Read the model definition and answer for the solid it produces. Units are mm, in the model's axes. A direction names the side the tool comes from. Give positions to 0.01 mm unless a question says otherwise; leave off trailing zeros. Loops run counter-clockwise (first coordinate to the right, second up) from the corner with the lowest first, then second, coordinate; pieces in that order, holes last.
(1) Straight lines are drawn through the part: probe 1 along X at (y, z) = (-58, 23); probe 2 along Z at (x, y) = (-60.5, -30); probe 3 along X at (y, z) = (15, 36.5). For each, find the intervals that lie inside material, in ascending order.
(2) Each of these flat-tipped pins is pushed along its axis until it touches: P1, Ø20, axis at x = -39.5, y = 27.5, coming from the +Z side; P2, Ø16, axis at y = -70.33, z = 27, coming from the -X side; P3, Ø16, axis at y = -67.5, z = 33, coming from the +X side; P4, Ø20, axis at x = -39, y = 23, coming from the -Z side. Where does it stop, or does it pass through?
(3) Find section D-D, the plane y = 10. Write down the section's boundary in (x, z), then the cut area to 3 significant figures.
(4) Find section B-B, the plane y = -39.5. Write down the section's boundary in (x, z).
(5) Which of the six approach directions +Z, -Z, +X, -X, +Y, -Y give full straight-line access (tool end or side, diameter ignored) to faces 1 (the face through (-24.833, 28, 27)), 2 (the face through (-38, 28, 14.5)), 3 (the face through (-38, 28, 39.5)), 4 (the face through (-34, 42.667, 18)), 5 (the face through (-49.833, 28, 27))?
(6) Find section C-C, the plane z = 50.5. Write down the section's boundary in (x, y).
(7) Find section A-A, the plane z = 27. State how many separate pieces and enclosed holes the cut face has, then the cut area to 3 significant figures.
```python
from build123d import *

# Parameters (mm, degrees)
SKETCH1_W           = 56
SKETCH1_H           = 140
BOSS_EXTRUDE1_DEPTH = 54
CUT_EXTRUDE4_DEPTH  = 54
SKETCH5_OUTSIDE_W   = 88.032
SKETCH5_OUTSIDE_H   = 174.032
SKETCH5_OUTSIDE_R   = 9
CUT_EXTRUDE6_DEPTH  = 60
SKETCH6_OUTSIDE_W   = 90.032
SKETCH6_OUTSIDE_H   = 88.032
SKETCH6_OUTSIDE_W_2 = 25
SKETCH6_OUTSIDE_H_2 = 25
CUT_EXTRUDE7_DEPTH  = 30
SKETCH7_R           = 9
BOSS_EXTRUDE2_DEPTH = 20


with BuildPart() as part:
    # Sketch1 → Boss-Extrude1 (new body)
    with BuildSketch(Plane.XY):
        with Locations((-37.333333333, -27.333333333)):
            Rectangle(SKETCH1_W, SKETCH1_H)
    extrude(amount=BOSS_EXTRUDE1_DEPTH)

    # Sketch2 → Cut-Extrude4 (cut)
    with BuildSketch(Plane.XY.offset(54)):
        with BuildLine():
            Line((-52.333333333, 6.259015594), (-52.333333333, 42.666666667))
            Line((-52.333333333, 42.666666667), (-65.333333333, 42.666666667))
            Line((-65.333333333, 42.666666667), (-65.333333333, -30.333333244))
            ThreePointArc((-65.333333333, -30.333333244), (-63.717759237, -20.959856403), (-59.057471264, -12.668061438))
            ThreePointArc((-59.057471264, -12.668061438), (-54.064305564, -3.783995357), (-52.333333333, 6.259015594))
        make_face()
        with BuildLine():
            Line((-37.333333333, -97.333333333), (-37.333333333, -18.333333333))
            ThreePointArc((-37.333333333, -18.333333333), (-47.23282827, -22.433838397), (-51.333333333, -32.333333333))
            Line((-51.333333333, -32.333333333), (-51.333333333, -54.582044639))
            Line((-51.333333333, -54.582044639), (-51.333333333, -97.333333333))
            Line((-51.333333333, -97.333333333), (-37.333333333, -97.333333333))
        make_face()
        with BuildLine():
            ThreePointArc((-37.333333333, -18.333333333), (-27.433838397, -22.433838397), (-23.333333333, -32.333333333))
            Line((-23.333333333, -32.333333333), (-23.333333333, -97.333333333))
            Line((-23.333333333, -97.333333333), (-9.333333333, -97.333333333))
            Line((-9.333333333, -97.333333333), (-9.333333333, 42.666666667))
            Line((-9.333333333, 42.666666667), (-22.333333333, 42.666666667))
            Line((-22.333333333, 42.666666667), (-37.333333333, 42.666666667))
            Line((-37.333333333, 42.666666667), (-37.333333333, -18.333333333))
        make_face()
        with BuildLine():
            Line((-23.333333333, -97.333333333), (-23.333333333, -32.333333333))
            ThreePointArc((-23.333333333, -32.333333333), (-27.433838397, -22.433838397), (-37.333333333, -18.333333333))
            Line((-37.333333333, -18.333333333), (-37.333333333, -97.333333333))
            Line((-37.333333333, -97.333333333), (-23.333333333, -97.333333333))
        make_face()
    extrude(amount=-CUT_EXTRUDE4_DEPTH, mode=Mode.SUBTRACT)

    # Mirror3: part across plane


with BuildPart() as part_1:
    add(part.part)
    add(part.part.mirror(Plane.ZY.offset(37.333333333)))

    # Sketch5 outside → Cut-Extrude6 (cut)
    # profile 1 of 2: a face of its own
    with BuildSketch(Plane(origin=(-9.333333333, 0, 0), x_dir=(0, 0, -1), z_dir=(1, 0, 0))):
        with Locations((-27, -27.333)):
            Rectangle(SKETCH5_OUTSIDE_W, SKETCH5_OUTSIDE_H)
        with BuildLine():
            Line((-42, 42.666666667), (-12, 42.666666667))
            Line((-12, 42.666666667), (-12, -35.347621964))
            ThreePointArc((-12, -35.347621964), (-10.377159088, -45.080907232), (-5.684210526, -53.761154264))
            ThreePointArc((-5.684210526, -53.761154264), (-27, -97.333333333), (-48.315789474, -53.761154264))
            ThreePointArc((-48.315789474, -53.761154264), (-43.622840912, -45.080907232), (-42, -35.347621964))
            Line((-42, -35.347621964), (-42, 42.666666667))
        make_face(mode=Mode.SUBTRACT)
    # profile 2 of 2: a face of its own
    with BuildSketch(Plane(origin=(-9.333333333, 0, 0), x_dir=(0, 0, -1), z_dir=(1, 0, 0))):
        with Locations(Location((-27, -70.333333333, 0), (0, 0, 90))):
            Circle(SKETCH5_OUTSIDE_R)
    extrude(amount=-CUT_EXTRUDE6_DEPTH, mode=Mode.SUBTRACT)

    # Sketch6 outside → Cut-Extrude7 (cut)
    with BuildSketch(Plane(origin=(0, 42.666666667, 0), x_dir=(1, 0, 0), z_dir=(0, 1, 0))):
        with Locations((-37.333, -27)):
            Rectangle(SKETCH6_OUTSIDE_W, SKETCH6_OUTSIDE_H)
        with Locations((-37.333333333, -27)):
            Rectangle(SKETCH6_OUTSIDE_W_2, SKETCH6_OUTSIDE_H_2, mode=Mode.SUBTRACT)
    extrude(amount=-CUT_EXTRUDE7_DEPTH, mode=Mode.SUBTRACT)

    # Sketch7 → Boss-Extrude2 (add)
    with BuildSketch(Plane(origin=(0, 42.666666667, 0), x_dir=(1, 0, 0), z_dir=(0, 1, 0))):
        with Locations(Location((-37.333333333, -27, 0), (0, 0, 270))):
            Circle(SKETCH7_R)
    extrude(amount=BOSS_EXTRUDE2_DEPTH)


solid = part_1.part
```
Entries:
1. probe 1: x = -65.33 to -51.33, -23.33 to -9.33
1. probe 2: z = 12 to 42
1. probe 3: x = -49.83 to -24.83
2. P1: stops at z = 39.5
2. P2: passes through
2. P3: stops at x = -9.33
2. P4: stops at z = 14.5
3. outline: (-52.33, 12) - (-22.33, 12) - (-22.33, 42) - (-52.33, 42) - close
3. area: 900 mm2
4. outline: (-65.33, 11.71) - (-51.33, 11.71) - (-51.33, 42.29) - (-65.33, 42.29) - close; (-23.33, 11.71) - (-9.33, 11.71) - (-9.33, 42.29) - (-23.33, 42.29) - close
5. face 1: +Z, -Z, +X, +Y
5. face 2: -Z, +X, -X, +Y
5. face 3: +Z, +X, -X, +Y
5. face 4: +Y
5. face 5: +Z, -Z, -X, +Y
6. outline: (-65.33, -83.63) - (-51.33, -83.63) - (-51.33, -57.04) - (-65.33, -57.04) - close; (-23.33, -83.63) - (-9.33, -83.63) - (-9.33, -57.04) - (-23.33, -57.04) - close
7. separate pieces: 3
7. enclosed holes: 0
7. area: 3,990 mm2
